The listing builds one solid part. Answer for the finished solid, in the listing's coordinates (mm). A direction names the side the tool comes from. Give positions to 0.01 mm unless a question says otherwise; leave off trailing zeros. Write each loop counter-clockwise with the first axis right and the second up, starting at its lowest first coordinate (ties: lowest second). Pieces come first, ordered by that corner, then holes.
```python
from build123d import *

# Parameters (mm, degrees)
SKETCH1_R           = 12.5
BOSS_EXTRUDE2_DEPTH = 12
SKETCH1_5_R         = 11.25
CUT_EXTRUDE1_DEPTH  = 10
CUT_EXTRUDE2_REACH  = 14
SKETCH4_R           = 1.5
BOSS_EXTRUDE3_DEPTH = 12
SKETCH11_W          = 8
SKETCH11_H          = 10
CUT_EXTRUDE6_DEPTH  = 10
SKETCH12_R          = 2
CUT_EXTRUDE7_DEPTH  = 14
SKETCH13_R          = 2
CUT_EXTRUDE8_DEPTH  = 14
SKETCH14_R          = 12.5
SKETCH14_R_2        = 11.25
BOSS_EXTRUDE4_DEPTH = 10


with BuildPart() as part:
    # Sketch1 → Boss-Extrude2 (new body)
    with BuildSketch(Plane.XY):
        Circle(SKETCH1_R)
    extrude(amount=BOSS_EXTRUDE2_DEPTH)

    # Sketch1<5> → Cut-Extrude1 (cut)
    with BuildSketch(Plane.XY):
        Circle(SKETCH1_5_R)
    extrude(amount=CUT_EXTRUDE1_DEPTH, mode=Mode.SUBTRACT)

    # Sketch4 → Cut-Extrude2 (cut, up to next)
    with BuildSketch(Plane.XY.offset(12), mode=Mode.PRIVATE) as cut_extrude2_sk1:
        with Locations((5.303300859, 5.303300859)):
            Circle(SKETCH4_R)
    cut_extrude2_tool1 = extrude(cut_extrude2_sk1.sketch, amount=-CUT_EXTRUDE2_REACH, mode=Mode.PRIVATE) & part.part
    add(cut_extrude2_tool1.solids().sort_by_distance((5.303301, 5.303301, 12))[0], mode=Mode.SUBTRACT)
    # Sketch4 → Cut-Extrude2 (cut, up to next)
    with BuildSketch(Plane.XY.offset(12), mode=Mode.PRIVATE) as cut_extrude2_sk2:
        with Locations((-5.303300859, 5.303300859)):
            Circle(SKETCH4_R)
    cut_extrude2_tool2 = extrude(cut_extrude2_sk2.sketch, amount=-CUT_EXTRUDE2_REACH, mode=Mode.PRIVATE) & part.part
    add(cut_extrude2_tool2.solids().sort_by_distance((-5.303301, 5.303301, 12))[0], mode=Mode.SUBTRACT)
    # Sketch4 → Cut-Extrude2 (cut, up to next)
    with BuildSketch(Plane.XY.offset(12), mode=Mode.PRIVATE) as cut_extrude2_sk3:
        with Locations((-5.303300859, -5.303300859)):
            Circle(SKETCH4_R)
    cut_extrude2_tool3 = extrude(cut_extrude2_sk3.sketch, amount=-CUT_EXTRUDE2_REACH, mode=Mode.PRIVATE) & part.part
    add(cut_extrude2_tool3.solids().sort_by_distance((-5.303301, -5.303301, 12))[0], mode=Mode.SUBTRACT)
    # Sketch4 → Cut-Extrude2 (cut, up to next)
    with BuildSketch(Plane.XY.offset(12), mode=Mode.PRIVATE) as cut_extrude2_sk4:
        with Locations((5.303300859, -5.303300859)):
            Circle(SKETCH4_R)
    cut_extrude2_tool4 = extrude(cut_extrude2_sk4.sketch, amount=-CUT_EXTRUDE2_REACH, mode=Mode.PRIVATE) & part.part
    add(cut_extrude2_tool4.solids().sort_by_distance((5.303301, -5.303301, 12))[0], mode=Mode.SUBTRACT)

    # Sketch10 → Boss-Extrude3 (add)
    with BuildSketch(Plane.XY):
        with BuildLine():
            Line((18.87387232, -13.229774891), (8.670952565, -9.003587153))
            ThreePointArc((8.670952565, -9.003587153), (12.259311424, -2.441164357), (11.458506302, 4.995261088))
            Line((11.458506302, 4.995261088), (24.231440373, -0.295461436))
            Line((24.231440373, -0.295461436), (20.787289482, -8.610377228))
            Line((20.787289482, -8.610377228), (18.87387232, -13.229774891))
        make_face()
        with BuildLine():
            Line((-24.231440373, -0.295461436), (-11.458506302, 4.995261088))
            ThreePointArc((-11.458506302, 4.995261088), (-12.259311424, -2.441164357), (-8.670952565, -9.003587153))
            Line((-8.670952565, -9.003587153), (-18.87387232, -13.229774891))
            Line((-18.87387232, -13.229774891), (-20.787289482, -8.610377228))
            Line((-20.787289482, -8.610377228), (-24.231440373, -0.295461436))
        make_face()
    extrude(amount=BOSS_EXTRUDE3_DEPTH)

    # Sketch11 → Cut-Extrude6 (cut)
    with BuildSketch(Plane(origin=(20.787289482, -8.610377228, 0), x_dir=(0, 0, -1), z_dir=(0.923879533, -0.382683432, 0))):
        with Locations((-6, 2)):
            Rectangle(SKETCH11_W, SKETCH11_H)
    cut_extrude6 = extrude(amount=-CUT_EXTRUDE6_DEPTH, mode=Mode.SUBTRACT)

    # Sketch12 → Cut-Extrude7 (cut)
    with BuildSketch(Plane(origin=(3.444150891, 8.314915793, 0), x_dir=(0.923879533, -0.382683432, 0), z_dir=(0.382683432, 0.923879533, 0))):
        with Locations((15.587337893, -6)):
            Circle(SKETCH12_R)
    extrude(amount=-CUT_EXTRUDE7_DEPTH, mode=Mode.SUBTRACT)

    # Mirror5: Cut-Extrude6 across plane
    add(cut_extrude6.mirror(Plane(origin=(0, 0, 0), x_dir=(0, 0, 1), z_dir=(1, 0, 0))), mode=Mode.SUBTRACT)

    # Sketch13 → Cut-Extrude8 (cut)
    with BuildSketch(Plane(origin=(-3.444150891, 8.314915793, 0), x_dir=(0.923879533, 0.382683432, 0), z_dir=(-0.382683432, 0.923879533, 0))):
        with Locations((-15.587337893, -6)):
            Circle(SKETCH13_R)
    extrude(amount=-CUT_EXTRUDE8_DEPTH, mode=Mode.SUBTRACT)

    # Sketch14 → Boss-Extrude4 (add)
    with BuildSketch(Plane(origin=(0, 0, 0), x_dir=(-1, 0, 0), z_dir=(0, 0, -1))):
        Circle(SKETCH14_R)
        Circle(SKETCH14_R_2, mode=Mode.SUBTRACT)
    extrude(amount=BOSS_EXTRUDE4_DEPTH)


solid = part.part
```
Item 1: A cutting plane is placed at B-B, the plane y = 10.75. Give the vertices of the cut face in (x, z).
Conclusion:
outline: (-6.38, -10) - (-3.32, -10) - (-3.32, 10) - (3.32, 10) - (3.32, -10) - (6.38, -10) - (6.38, 12) - (-6.38, 12) - close
Item 2: A cutting plane is placed at A-A, the plane x = 0. Give the vertices of the cut face in (y, z).
Conclusion:
outline: (-12.5, -10) - (-11.25, -10) - (-11.25, 10) - (11.25, 10) - (11.25, -10) - (12.5, -10) - (12.5, 12) - (-12.5, 12) - close
Item 3: Each of these flat-tipped pins is pushed along its axis until it touches: P1, Ø1, axis at y = 10, z = 0, coming from the +X side; P2, Ø7, axis at x = 4, y = -3.5, coming from the -Z side; P3, Ø1.5, axis at y = -3, z = -4.5, coming from the -X side; P4, Ø2.5, axis at x = -5.3, y = 5.3, coming from the +Z side. Where does it stop, or does it pass through?
Conclusion:
P1: stops at x = 8.12
P2: stops at z = 10
P3: stops at x = -12.3
P4: passes through
Item 4: A cutting plane is placed at D-D, the plane y = 0.5. Count the separate pieces of the cut face and the enclosed holes in it, plus the area to 3 significant figures.
Conclusion:
separate pieces: 1
enclosed holes: 2
area: 269 mm2
Item 5: A cutting plane is placed at C-C, the plane z = -6. Give the vertices of the cut face in (x, y), plus the area to 3 significant figures.
Conclusion:
outline: circle Ø25 at (0, 0); hole circle Ø22.5 at (0, 0)
area: 93.3 mm2
Item 6: Determine the mould class of faces 1 (the face through (-16.615, 1.792, 7.774)), 2 (the face through (0, -3, 12)), 3 (the face through (16.336, 2.975, 4.583)) for opening direction X: pulls with the +X half, pulls with the -X half, needs draft (parallel to the pull), parting line crosses it, or undercut.
Conclusion:
face 1: undercut
face 2: needs draft
face 3: pulls with the +X half
Item 7: Which of the six approach directions +Z, -Z, +X, -X, +Y, -Y give full straight-line access (tool end or side, diameter ignored) to faces 4 (the face through (-17, -5, 10)), 5 (the face through (-14.835, -11.557, 5.916)), 6 (the face through (-16.11, -9.92, 6.06)), 7 (the face through (0, 0, 10))?
Conclusion:
face 4: none
face 5: +Z, -Z, -Y
face 6: -X
face 7: -Z
Item 8: Consider probe 1 along X at (y, z) = (0, -5.25); probe 2 along Y at (x, z) = (4, 10.25); probe 3 along X at (y, z) = (-9.25, 4.25). Determine where each line is inside the solid, lowest interval first.
Conclusion:
probe 1: x = -12.5 to -11.25, 11.25 to 12.5
probe 2: y = -11.84 to -6.05, -4.56 to 4.56, 6.05 to 11.84
probe 3: x = -14.49 to -14.09, -11.99 to -9.27, -8.41 to -6.4, 6.4 to 8.41, 9.27 to 11.99, 14.09 to 14.49
